```python
from build123d import *

# Parameters (mm, degrees)
CUT_EXTRUDE1_DEPTH      = 9.844526556
CUT_EXTRUDE1_DEPTH_BACK = 9.844526556
SKETCH2_R               = 2.54
SKETCH3_R               = 3.175
CUT_EXTRUDE2_DEPTH      = 5.08


with BuildPart() as part:
    # Sketch1 → Revolve1 (revolve)
    with BuildSketch(Plane(origin=(0, 0, 0), x_dir=(1, 0, 0), z_dir=(0, 1, 0))):
        with BuildLine():
            Line((0, 3.175), (0, -3.175))
            ThreePointArc((0, -3.175), (-3.175, 0), (0, 3.175))
        make_face()
    revolve(axis=Axis((0, 0, -3.175), (0, 0, 1)))

    # Sketch2 → Cut-Extrude1 (cut, two sides: drawn at the far end of the back side and taken through both)
    with BuildSketch(Plane(origin=(4.445, 0, 0), x_dir=(0, 0, -1), z_dir=(1, 0, 0)).offset(-CUT_EXTRUDE1_DEPTH_BACK)):
        Circle(SKETCH2_R)
    extrude(amount=CUT_EXTRUDE1_DEPTH + CUT_EXTRUDE1_DEPTH_BACK, mode=Mode.SUBTRACT)

    # Sketch3 → Cut-Extrude2 (cut)
    with BuildSketch(Plane(origin=(6.35, 0, 0), x_dir=(0, 0, -1), z_dir=(1, 0, 0))):
        Circle(SKETCH3_R)
    cut_extrude2 = extrude(amount=-CUT_EXTRUDE2_DEPTH, mode=Mode.SUBTRACT)

    # Mirror1: Cut-Extrude2 across plane
    add(cut_extrude2.mirror(Plane(origin=(0, 0, 0), x_dir=(0, 0, 1), z_dir=(1, 0, 0))), mode=Mode.SUBTRACT)


solid = part.part
```
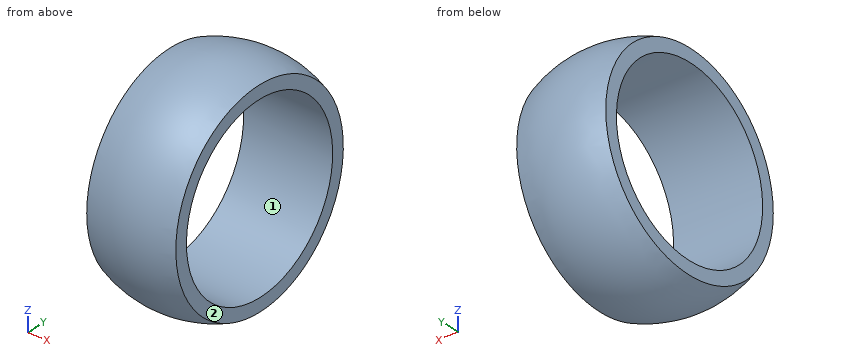
Geometry check sheet. Reference: the model listing, model coordinates, mm. Face numbers are marked on the shaded views. Give positions to 0.01 mm unless a question says otherwise; leave off trailing zeros. Write each loop counter-clockwise with the first axis right and the second up, starting at its lowest first coordinate (ties: lowest second). Pieces come first, ordered by that corner, then holes.
1) Release check for a two-part mould opening along Z. For the marked faces 1 and 2 record: pulls with the +Z half, pulls with the -Z half, needs draft (parallel to the pull), parting line crosses it, or undercut.
2) Section check A-A, the plane y = 0. Record the boundary of the cut face in (x, z) (3 decimals), and give its area (3 significant figures).
3) Section check D-D, the plane x = -0.9. Record the boundary of the cut face in (y, z).
4) Gauge pin test, flat end, axial feed: pin 1 (1.5 mm diameter, centred on x = 1, z = 1, fed in from -Y). Record the tip position at first contact, or that the pin passes through.
5) Material ranges on L1, parallel to Z at x = 0.05, y = 0; L2, parallel to Z at x = -0.45, y = 0.75; L3, parallel to Y at x = -0.9, z = 1, recorded low to high.
6) Section check C-C, the plane x = 0.7. Record the boundary of the cut face in (y, z), and give its area (3 significant figures).
Computed:
1. face 1: undercut
1. face 2: needs draft
2. outline: (-1.27, -2.91) arc R3.175 ccw to (1.27, -2.91) - (1.27, -2.54) - (-1.27, -2.54) - close; (-1.27, 2.54) - (1.27, 2.54) - (1.27, 2.91) arc R3.175 ccw to (-1.27, 2.91) - close
2. area: 2.78 mm2
3. outline: circle Ø6.09 at (0, 0); hole circle Ø5.08 at (0, 0)
4. pin 1: stops at y = -3.1
5. L1: z = -3.17 to -2.54, 2.54 to 3.17
5. L2: z = -3.05 to -2.43, 2.43 to 3.05
5. L3: y = -2.88 to -2.33, 2.33 to 2.88
6. outline: circle Ø6.19 at (0, 0); hole circle Ø5.08 at (0, 0)
6. area: 9.86 mm2
